```python
from build123d import *

# Parameters (mm, degrees)
F0_W     = 664.733171463
F0_H     = 712.0994329453
F1_DEPTH = 431.8
F2_T     = -25.4
F3_W     = 613.933171463
F3_H     = 194.4507785797
F4_DEPTH = 25.4
F5_W     = 401.3557694852
F5_H     = 468.805462122
F6_DEPTH = 25.4
F7_W     = 392.9471150041
F7_H     = 457.1952670813
F8_DEPTH = 25.4
F9_DEPTH = 10.668


with BuildPart() as f1:
    # F0 (on Front) → F1 (new body)
    with BuildSketch(Plane.XZ):
        Rectangle(F0_W, F0_H)
    extrude(amount=F1_DEPTH)

    # F2
    f2_openings = [f1.faces().sort_by_distance(p)[0] for p in [
        (0, -431.8, 0),
    ]]
    offset(amount=F2_T, openings=f2_openings)

    # F3 (on face) → F4 (join)
    with BuildSketch(Plane.XZ.offset(431.8)):
        with Locations((0, -233.4243271828)):
            Rectangle(F3_W, F3_H)
    extrude(amount=-F4_DEPTH)

    # F5 (on face) → F6 (cut)
    with BuildSketch(Plane.YZ.offset(332.3665857315)):
        with Locations((-217.3207271844, 89.9267345667)):
            Rectangle(F5_W, F5_H)
    extrude(amount=-F6_DEPTH, mode=Mode.SUBTRACT)

    # F7 (on face) → F8 (cut)
    with BuildSketch(Plane(origin=(-332.3665857315, 0, 0), x_dir=(0, -1, 0), z_dir=(-1, 0, 0))):
        with Locations((217.2129563987, 94.2879095674)):
            Rectangle(F7_W, F7_H)
    extrude(amount=-F8_DEPTH, mode=Mode.SUBTRACT)

    # F9 (add): a face of the model
    f9_faces = [f1.faces().sort_by_distance(p)[0] for p in [
        (319.6665857315, -217.3207271844, -144.4759964943),
    ]]
    extrude(f9_faces, amount=F9_DEPTH)


solid = f1.part
```
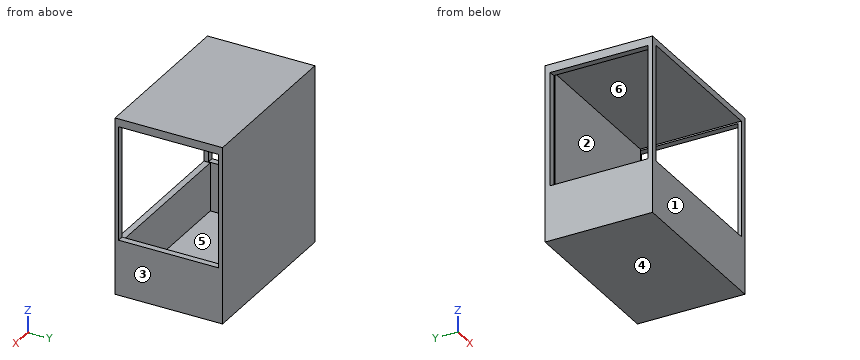
Work out the finished part from the listing and answer in its coordinate system (mm). Face numbers are marked on the shaded views. A direction names the side the tool comes from. Round coordinates to 2 decimals unless told otherwise and drop trailing zeros. Loops run counter-clockwise (first coordinate to the right, second up) from the corner with the lowest first, then second, coordinate; pieces in that order, holes last. Notation, with made-up numbers: (34, 88) -> (45, 88) arc R15 ccw to (45, 92) -> close; hole circle Ø8 at (14, 26.25). An arc over 180 degrees is marked (long way). Write each question's results on one line, items separated by ' | '. Start each with the question number.
1. Section A-A (y = -170) is taken. Determine the outline of the cut face in (x, z).
2. Section D-D (x = 167.5) is taken. Determine the outline of the cut face in (y, z).
3. Section C-C (z = -214.5) is taken. Determine the outline of the cut face in (x, y), plus the area to 3 significant figures.
4. A tool of negligible diameter and unlimited length cuts with its end or side. For the marked faces 4, 5 and 6, from which of +Z, -Z, +X, -X, +Y, -Y can it reach the whole face along a straight path? Write none if from no direction.
5. Given pin 1 Ø12.5 at (x, z) = (317.5, 7) entering from +Y; pin 2 Ø6 at (x, z) = (43.5, -93) entering from -Y, each flat-ended and moving along its own axis, determine where each tip first touches the part or whether it passes through.
6. Find the intervals of material crossed by probe 1 along Z at (x, y) = (-20, -216); probe 2 along X at (y, z) = (-232, -177.5); probe 3 along Y at (x, z) = (-75.5, -273.5), in increasing order. Write a range as from..to.
7. For a pull along Y with two mould halves and no side action, classify the marked faces 1, 2 and 3 as +Y half, -Y half, draft (parallel to the pull), parting line (faces both ways), or undercut.
8. Section B-B (z = 109.5) is taken. Determine the outline of the cut face in (x, y), plus the area to 3 significant figures.
Evaluation:
1) outline: (-332.37, -356.05) -> (332.37, -356.05) -> (332.37, -133.81) -> (306.97, -133.81) -> (306.97, -330.65) -> (-306.97, -330.65) -> (-306.97, -134.31) -> (-332.37, -134.31) -> close; (-332.37, 322.89) -> (-306.97, 322.89) -> (-306.97, 330.65) -> (306.97, 330.65) -> (306.97, 324.33) -> (332.37, 324.33) -> (332.37, 356.05) -> (-332.37, 356.05) -> close
2) outline: (-431.8, -356.05) -> (0, -356.05) -> (0, 356.05) -> (-431.8, 356.05) -> (-431.8, 330.65) -> (-25.4, 330.65) -> (-25.4, -330.65) -> (-406.4, -330.65) -> (-406.4, -136.2) -> (-431.8, -136.2) -> close
3) outline: (-332.37, -431.8) -> (332.37, -431.8) -> (332.37, 0) -> (-332.37, 0) -> close; hole (-306.97, -406.4) -> (306.97, -406.4) -> (306.97, -25.4) -> (-306.97, -25.4) -> close | area: 53,100 mm2
4) face 4: -Z, +X, -X, +Y, -Y | face 5: none | face 6: -Y
5) pin 1: stops at y = 0 | pin 2: stops at y = -25.4
6) probe 1: z = -356.05..-330.65, 330.65..356.05 | probe 2: x = -332.37..-306.97, 306.97..332.37 | probe 3: y = -431.8..-406.4, -25.4..0
7) face 1: -Y half | face 2: undercut | face 3: draft
8) outline: (-332.37, -431.8) -> (-306.97, -431.8) -> (-306.97, -413.69) -> (-332.37, -413.69) -> close; (-332.37, -20.74) -> (-306.97, -20.74) -> (-306.97, -25.4) -> (306.97, -25.4) -> (306.97, -16.64) -> (332.37, -16.64) -> (332.37, 0) -> (-332.37, 0) -> close; (306.97, -431.8) -> (332.37, -431.8) -> (332.37, -418) -> (306.97, -418) -> close | area: 17,400 mm2
